```python
from build123d import *

# Parameters (mm, degrees)
BOSS_EXTRU_1_DEPTH      = 6
ESQUISSE2_W             = 181
ESQUISSE2_H             = 61
ENL_V_MAT_EXTRU_1_DEPTH = 314.10221973
ESQUISSE4_R             = 1.5
ESQUISSE4_R_2           = 2.037365752
ENL_V_MAT_EXTRU_2_DEPTH = 314.10221973
ESQUISSE5_R             = 2.995
ENL_V_MAT_EXTRU_3_DEPTH = 3


with BuildPart() as part:
    # Esquisse1 → Boss.-Extru.1 (new body)
    with BuildSketch(Plane.XY):
        Polygon((-301, 80), (-281, 80), (-281, 86), (-261, 86), (-261, 80), (-40, 80), (-40, 86), (-20, 86), (-20, 80), (0, 80), (0, 0), (-20, 0), (-20, -6), (-40, -6), (-40, 0), (-140.5, 0), (-140.5, -6), (-160.5, -6), (-160.5, 0), (-261, 0), (-261, -6), (-281, -6), (-281, 0), (-301, 0), align=None)
    extrude(amount=BOSS_EXTRU_1_DEPTH)

    # Esquisse2 → Enlèv. mat.-Extru.1 (cut, through all)
    with BuildSketch(Plane.XY.offset(6)):
        with Locations((-150.5, 49.5)):
            Rectangle(ESQUISSE2_W, ESQUISSE2_H)
    extrude(amount=-ENL_V_MAT_EXTRU_1_DEPTH, mode=Mode.SUBTRACT)

    # Esquisse4 → Enlèv. mat.-Extru.2 (cut, through all)
    with BuildSketch(Plane.XY.offset(6)):
        with Locations((-271, 83)):
            Circle(ESQUISSE4_R)
        with Locations((-30, 83)):
            Circle(ESQUISSE4_R)
        with Locations(Location((-30, -3, 0), (0, 0, 180))):
            Circle(ESQUISSE4_R)
        with Locations(Location((-271, -3, 0), (0, 0, 180))):
            Circle(ESQUISSE4_R)
        with Locations((-150.5, -3)):
            Circle(ESQUISSE4_R_2)
    extrude(amount=-ENL_V_MAT_EXTRU_2_DEPTH, mode=Mode.SUBTRACT)

    # Esquisse5 → Enlèv. mat.-Extru.3 (cut)
    with BuildSketch(Plane.XY.offset(6)):
        with Locations((-271, 83)):
            Circle(ESQUISSE5_R)
        with Locations((-30, 83)):
            Circle(ESQUISSE5_R)
        with Locations((-271, -3)):
            Circle(ESQUISSE5_R)
        with Locations((-150.5, -3)):
            Circle(ESQUISSE5_R)
        with Locations((-30, -3)):
            Circle(ESQUISSE5_R)
    extrude(amount=-ENL_V_MAT_EXTRU_3_DEPTH, mode=Mode.SUBTRACT)


solid = part.part
```
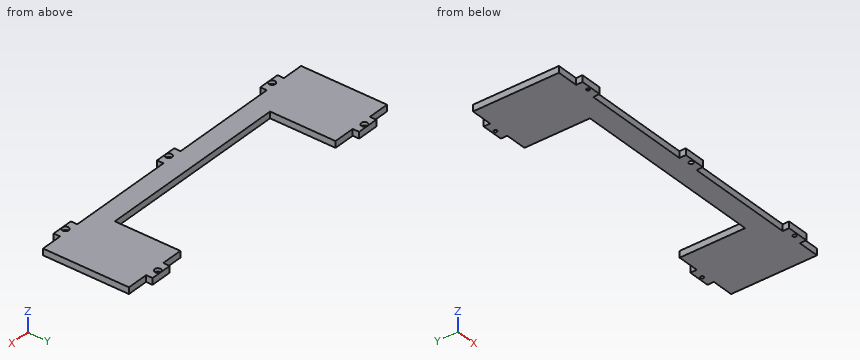
Could you check a few things on this model? Use its own coordinates, in mm. Coordinates: 2 decimals unless noted, no trailing zeros. Write each loop counter-clockwise with the first axis right and the second up, starting at its lowest first coordinate (ties: lowest second). Pieces come first, ordered by that corner, then holes. Notation, with made-up numbers: (4, 5.25) -> (43, 5.25) arc R35 ccw to (43, 43.25) -> close; hole circle Ø4 at (89.5, 35.5). An arc over 180 degrees is marked (long way). One line per question, with ' | ' between items. Start each with the question number.
1. If we section it at C-C (x = -53): Please give me the cut outline in (y, z).
2. If we section it at A-A (y = 32.5): Please give me the cut outline in (x, z), and give its area (3 significant figures).
3. Will these pins go through, and if not, where does the flat tip stop? P1, Ø1.8, axis at x = -246, z = 3.5, coming from the +Y side; P2, Ø1, axis at x = -202, z = 3.5, coming from the -Y side; P3, Ø3, axis at y = 82, z = 3.5, coming from the -X side.
4. Please list where these lines run through material, in increasing order: line 1 along X through (y, z) = (83, 1.6); line 2 along Y through (x, z) = (-271, 1.5); line 3 along X through (y, z) = (38, 1.1).
5. If we section it at B-B (z = 1.65): Count the separate pieces of the cut face and the enclosed holes in it, and give its area (3 significant figures).
Return value:
1) outline: (0, 0) -> (80, 0) -> (80, 6) -> (0, 6) -> close
2) outline: (-301, 0) -> (-241, 0) -> (-241, 6) -> (-301, 6) -> close; (-60, 0) -> (0, 0) -> (0, 6) -> (-60, 6) -> close | area: 720 mm²
3) P1: stops at y = 80 | P2: stops at y = 0 | P3: stops at x = -281
4) line 1: x = -281 to -272.5, -269.5 to -261, -40 to -31.5, -28.5 to -20 | line 2: y = -6 to -4.5, -1.5 to 81.5, 84.5 to 86 | line 3: x = -301 to -241, -60 to 0
5) separate pieces: 1 | enclosed holes: 5 | area: 13,600 mm²
